Geometry check sheet. Reference: the model listing, model coordinates, mm. Face numbers are marked on the shaded views. A direction names the side the tool comes from. Give positions to 0.01 mm unless a question says otherwise; leave off trailing zeros. Order: outer loops, then holes, each group sorted by start corner. A loop starts at its lowest first (then second) coordinate and runs counter-clockwise, first axis right, second up.
```python
from build123d import *

# Parameters (mm, degrees)
SKETCH5_W          = 17.5
SKETCH5_H          = 13.5
CUT_EXTRUDE1_DEPTH = 6.35
SKETCH6_W          = 17.5
SKETCH6_H          = 2.032
CUT_EXTRUDE2_DEPTH = 10.16


with BuildPart() as part:
    # Sketch3 → Revolve1 (revolve)
    with BuildSketch(Plane.XY):
        Polygon((17.5, 0), (1.27, 5.442857143), (1.27, 6.858), (21.5, 6.858), (21.5, 0), align=None)
    revolve(axis=Axis((0, 0, 0), (0, -1, 0)))

    # Sketch5 → Cut-Extrude1 (cut)
    with BuildSketch(Plane(origin=(0, 12.7, 0), x_dir=(1, 0, 0), z_dir=(0, 1, 0))):
        with Locations((0, 0.75)):
            Rectangle(SKETCH5_W, SKETCH5_H)
    extrude(amount=-CUT_EXTRUDE1_DEPTH, mode=Mode.SUBTRACT)

    # Sketch6 → Cut-Extrude2 (cut)
    with BuildSketch(Plane(origin=(0, 15.24, 0), x_dir=(1, 0, 0), z_dir=(0, 1, 0))):
        with Locations((0, 5.2)):
            Rectangle(SKETCH6_W, SKETCH6_H)
    extrude(amount=-CUT_EXTRUDE2_DEPTH, mode=Mode.SUBTRACT)


solid = part.part
```
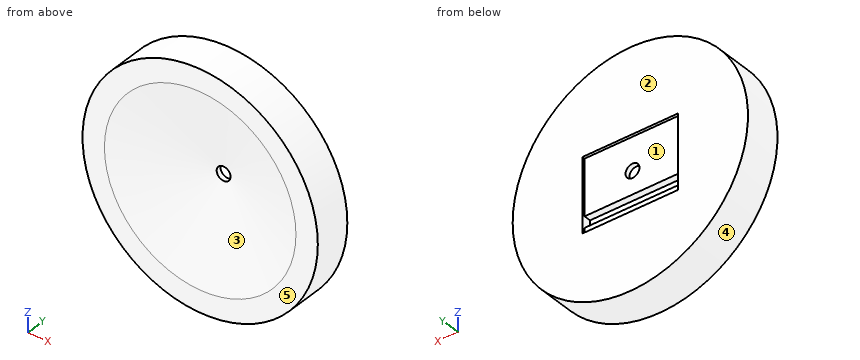
Q1. Gauge pin test, flat ends, axial feed: P1, Ø0.9, axis at y = 6, z = -3, coming from the +X side; P2, Ø6, axis at x = -1, z = 10, coming from the -Y side; P3, Ø1.5, axis at x = 10, y = 3, coming from the -Z side. Record the tip position at first contact, or that the pin passes through.
Q2. Cross-section at A-A, the plane x = 0. Record the boundary of the cut face in (y, z), and give its area (3 significant figures).
Q3. Cross-section at B-B, the plane z = 0. Record the boundary of the cut face in (x, y).
Q4. Release check for a two-part mould opening along X. For the marked faces 3, 4 and 5 record: pulls with the +X half, pulls with the -X half, needs draft (parallel to the pull), parting line crosses it, or undercut.
Q5. Thickness scan on L1, parallel to Z at x = 0, y = 6.25; L2, parallel to Z at x = -1.5, y = 5.75; L3, parallel to Z at x = -16, y = 5.75. Record the ranges inside material, lowest first.
Q6. Access from +Z, -Z, +X, -X, +Y, -Y to the whole of each face (thin tool, end or side, straight path). Record for the marked faces 1 and 2.
Q7. Cross-section at D-D, the plane x = -18. Record the boundary of the cut face in (y, z).
Q8. Cross-section at C-C, the plane y = 4. Record the boundary of the cut face in (x, z).
Answers follow:
1. P1: stops at x = 21.35
1. P2: stops at y = 1.49
1. P3: stops at z = -19.41
2. outline: (0, -21.5) - (6.86, -21.5) - (6.86, -7.5) - (6.35, -7.5) - (6.35, -6.22) - (5.08, -6.22) - (5.08, -4.18) - (6.35, -4.18) - (6.35, -1.27) - (5.44, -1.27) - (0, -17.5) - close; (0, 17.5) - (5.44, 1.27) - (6.35, 1.27) - (6.35, 6) - (6.86, 6) - (6.86, 21.5) - (0, 21.5) - close
2. area: 181 mm2
3. outline: (-21.5, 0) - (-17.5, 0) - (-1.27, 5.44) - (-1.27, 6.35) - (-8.75, 6.35) - (-8.75, 6.86) - (-21.5, 6.86) - close; (1.27, 5.44) - (17.5, 0) - (21.5, 0) - (21.5, 6.86) - (8.75, 6.86) - (8.75, 6.35) - (1.27, 6.35) - close
4. face 3: undercut
4. face 4: parting line crosses it
4. face 5: needs draft
5. L1: z = -21.5 to -6.22, -4.18 to -1.27, 1.27 to 21.5
5. L2: z = -21.45 to -6.22, -4.18 to 21.45
5. L3: z = -14.36 to 14.36
6. face 1: +Y
6. face 2: +Z, -Z, +X, -X, +Y
7. outline: (0, -11.76) - (6.86, -11.76) - (6.86, 11.76) - (0, 11.76) - close
8. outline: circle Ø43 at (0, 0); hole circle Ø11.14 at (0, 0)
